from build123d import *

# Parameters (mm, degrees)
SKETCH2_R                = 25
SKETCH2_R_2              = 10
BOSS_EXTRUDE1_DEPTH      = 295
BOSS_EXTRUDE2_DEPTH      = 310
BOSS_EXTRUDE2_DEPTH_BACK = 310
SKETCH2_3_R              = 10


with BuildPart() as part:
    # Sketch2 → Boss-Extrude1 (new, symmetric)
    # profile 1 of 2: a face of its own
    with BuildSketch(Plane.XY):
        Circle(SKETCH2_R)
        Circle(SKETCH2_R_2, mode=Mode.SUBTRACT)
    # profile 2 of 2: a face of its own
    with BuildSketch(Plane.XY):
        Circle(SKETCH2_R_2)
    extrude(amount=BOSS_EXTRUDE1_DEPTH, both=True)

    # Sketch2_3 → Boss-Extrude2 (add, two sides: drawn at the far end of the back side and taken through both)
    with BuildSketch(Plane.XY.offset(-BOSS_EXTRUDE2_DEPTH_BACK)):
        Circle(SKETCH2_3_R)
    extrude(amount=BOSS_EXTRUDE2_DEPTH + BOSS_EXTRUDE2_DEPTH_BACK)


solid = part.part
Could you check a few things on this model? Use its own coordinates, in mm. A direction names the side the tool comes from. Coordinates: 2 decimals unless noted, no trailing zeros. Loops run counter-clockwise (first coordinate to the right, second up) from the corner with the lowest first, then second, coordinate; pieces in that order, holes last. Notation, with made-up numbers: (-8, 45.25) -> (10, 45.25) arc R11 cw to (10, 66.25) -> close; hole circle Ø5 at (-20, 47.5). An arc over 180 degrees is marked (long way). Answer in a Markdown table with one row per item.
(1) Imagine slicing it at C-C (z = -53.5). List the corners of the cut face in (x, y) for me.
Results found:
| item | result |
|---|---|
| outline | circle Ø50 at (0, 0) |
(2) Will these pins go through, and if not, where does the flat tip stop? pin 1 Ø1.5 at (x, z) = (16, -61.5) entering from -Y; pin 2 Ø1 at (x, y) = (-16, 18.5) entering from -Z; pin 3 Ø5 at (y, z) = (18, -64.5) entering from +X.
Results found:
| item | result |
|---|---|
| pin 1 | stops at y = -19.81 |
| pin 2 | stops at z = -295 |
| pin 3 | stops at x = 19.62 |
(3) Imagine slicing it at A-A (y = 0). List the corners of the cut face in (x, z) for me.
Results found:
| item | result |
|---|---|
| outline | (-25, -295) -> (-10, -295) -> (-10, -310) -> (10, -310) -> (10, -295) -> (25, -295) -> (25, 295) -> (10, 295) -> (10, 310) -> (-10, 310) -> (-10, 295) -> (-25, 295) -> close |
(4) If I drill on probe 1 along X at (y, z) = (-1, -24); probe 2 along Z at (x, y) = (10.5, 10.5); probe 3 along Y at (x, z) = (1.5, 220), over which ranges is the centre line in solid material (lowest first)?
Results found:
| item | result |
|---|---|
| probe 1 | x = -24.98 to 24.98 |
| probe 2 | z = -295 to 295 |
| probe 3 | y = -24.95 to 24.95 |
(5) For faces 3 (the face through (0, -11, -295)), 4 (the face through (0, -11, 295)), 5 (the face through (0, 0, 310)), which set-ups out of +Z, -Z, +X, -X, +Y, -Y let a thin tool reach every point of the face, with its end or its side?
Results found:
| item | result |
|---|---|
| face 3 | -Z |
| face 4 | +Z |
| face 5 | +Z, +X, -X, +Y, -Y |
(6) Thinking about a two-plate mould opening in X: for faces 1 (the face through (-2.17, -9.76, -302.6)), 2 (the face through (0, 0, -310)), which applies, released by +X, released by -X, zero draft, split by the parting line, or undercut?
Results found:
| item | result |
|---|---|
| face 1 | split by the parting line |
| face 2 | zero draft |
